from build123d import *

# Parameters (mm, degrees)
SKETCH1_R           = 2.25
SKETCH1_R_2         = 20
BOSS_EXTRUDE1_DEPTH = 6


with BuildPart() as part:
    # Sketch1 → Boss-Extrude1 (new body)
    with BuildSketch(Plane(origin=(0, 0, 0), x_dir=(1, 0, 0), z_dir=(0, 1, 0))):
        with BuildLine():
            Line((0, -25), (0, 25))
            ThreePointArc((0, 25), (1.464466094, 28.535533906), (5, 30))
            Line((5, 30), (95, 30))
            ThreePointArc((95, 30), (98.535533906, 28.535533906), (100, 25))
            Line((100, 25), (100, -25))
            ThreePointArc((100, -25), (98.535533906, -28.535533906), (95, -30))
            Line((95, -30), (5, -30))
            ThreePointArc((5, -30), (1.464466094, -28.535533906), (0, -25))
        make_face()
        with Locations(Location((95, 25, 0), (0, 0, 270))):
            Circle(SKETCH1_R, mode=Mode.SUBTRACT)
        with Locations(Location((45, 25, 0), (0, 0, 270))):
            Circle(SKETCH1_R, mode=Mode.SUBTRACT)
        with Locations(Location((45, -25, 0), (0, 0, 90))):
            Circle(SKETCH1_R, mode=Mode.SUBTRACT)
        with Locations(Location((95, -25, 0), (0, 0, 90))):
            Circle(SKETCH1_R, mode=Mode.SUBTRACT)
        with Locations(Location((70, 0, 0), (0, 0, 270))):
            Circle(SKETCH1_R_2, mode=Mode.SUBTRACT)
        with BuildLine():
            Line((10, 19), (30, 19))
            ThreePointArc((30, 19), (34, 15), (30, 11))
            Line((30, 11), (10, 11))
            ThreePointArc((10, 11), (6, 15), (10, 19))
        make_face(mode=Mode.SUBTRACT)
        with BuildLine():
            Line((10, -19), (30, -19))
            ThreePointArc((30, -19), (34, -15), (30, -11))
            Line((30, -11), (10, -11))
            ThreePointArc((10, -11), (6, -15), (10, -19))
        make_face(mode=Mode.SUBTRACT)
    extrude(amount=BOSS_EXTRUDE1_DEPTH)


solid = part.part
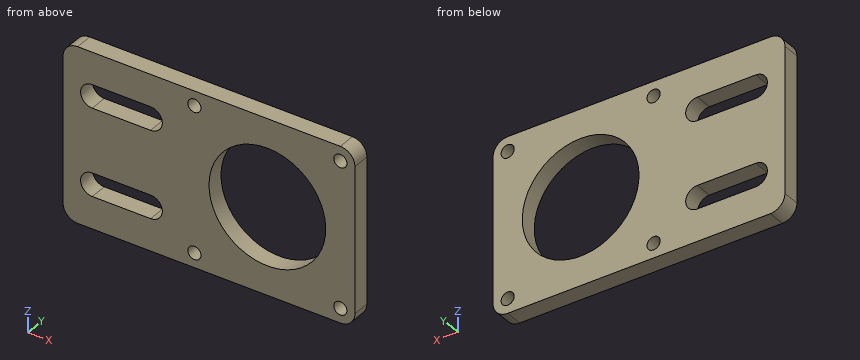
For this review, take the finished solid that the model builds, in its own axes (mm). Give positions to 0.01 mm unless a question says otherwise; leave off trailing zeros. Loops run counter-clockwise (first coordinate to the right, second up) from the corner with the lowest first, then second, coordinate; pieces in that order, holes last. Notation, with made-up numbers: (-14.75, 13) - (37.25, 13) arc R21 ccw to (37.25, 35) - close; hole circle Ø4 at (14.5, 88). An arc over 180 degrees is marked (long way). Write each question's results on one line, items separated by ' | '.
(1) For line 1 along Z through (x, y) = (25.5, 4.1); line 2 along X through (y, z) = (2.7, -11.5); line 3 along X through (y, z) = (0.7, 0), list the stretches that pass through material, from the lowest coordinate up.
Conclusion:
line 1: -30 to -19, -11 to 11, 19 to 30 | line 2: 0 to 8.06, 31.94 to 53.64, 86.36 to 100 | line 3: 0 to 50, 90 to 100
(2) Take a section at D-D (x = 70). Give the boundary of the cut face in (y, z), then the cut area to 3 significant figures.
Conclusion:
outline: (0, -30) - (6, -30) - (6, -20) - (0, -20) - close; (0, 20) - (6, 20) - (6, 30) - (0, 30) - close | area: 120 mm^2
(3) Take a section at A-A (x = 45). Give the boundary of the cut face in (y, z).
Conclusion:
outline: (0, -30) - (6, -30) - (6, -27.25) - (0, -27.25) - close; (0, -22.75) - (6, -22.75) - (6, 22.75) - (0, 22.75) - close; (0, 27.25) - (6, 27.25) - (6, 30) - (0, 30) - close
(4) Take a section at B-B (y = 3.25). Give the boundary of the cut face in (x, z).
Conclusion:
outline: (0, -25) arc R5 ccw to (5, -30) - (95, -30) arc R5 ccw to (100, -25) - (100, 25) arc R5 ccw to (95, 30) - (5, 30) arc R5 ccw to (0, 25) - close; hole (10, -19) - (30, -19) arc R4 ccw to (30, -11) - (10, -11) arc R4 ccw to start; hole (10, 11) - (30, 11) arc R4 ccw to (30, 19) - (10, 19) arc R4 ccw to start; hole circle Ø4.5 at (45, -25); hole circle Ø4.5 at (45, 25); hole circle Ø40 at (70, 0); hole circle Ø4.5 at (95, -25); hole circle Ø4.5 at (95, 25)
(5) For pin 1 Ø6 at (x, z) = (95, 25) entering from +Y, flat-tipped, find the tip position at first contact; note if it passes through.
Conclusion:
pin 1: y = 6
(6) Take a section at C-C (z = 0). Give the boundary of the cut face in (x, y), then the cut area to 3 significant figures.
Conclusion:
outline: (0, 0) - (50, 0) - (50, 6) - (0, 6) - close; (90, 0) - (100, 0) - (100, 6) - (90, 6) - close | area: 360 mm^2
